```python
from build123d import *

# Parameters (mm, degrees)
F1_DEPTH = 76.708
F2_DEPTH = 77.47
F3_DEPTH = 38.1


with BuildPart() as f1:
    # F0 (on Top) → F1 (new body)
    with BuildSketch(Plane.XY):
        Polygon((135.3836357594, 21.8498203903), (-49.6764220297, -59.8627962172), (146.1022645235, -72.4891498685), align=None)
    extrude(amount=F1_DEPTH)

    # F2 (add): a face of the model
    f2_faces = [f1.faces().sort_by_distance(p)[0] for p in [
        (140.7429501414, -25.3196647391, 38.354),
    ]]
    extrude(f2_faces, amount=F2_DEPTH)

    # F3 (add): a face of the model
    f3_faces = [f1.faces().sort_by_distance(p)[0] for p in [
        (122.6602477732, -29.7614131006, 76.708),
    ]]
    extrude(f3_faces, amount=F3_DEPTH)


solid = f1.part
```
Source: CAD feature listing. Evaluate the final solid. Frame: model axes, mm. Round coordinates to 2 decimals unless told otherwise and drop trailing zeros. Order: outer loops, then holes, each group sorted by start corner. A loop starts at its lowest first (then second) coordinate and runs counter-clockwise, first axis right, second up. Notation, with made-up numbers: (15, 47) -> (27, 47) arc R25 cw to (27, 82) -> close; hole circle Ø2 at (21, 38). An arc over 180 degrees is marked (long way). One line per item, written item: value. Start each with the question number.
Q1. Section query C-C (x = 33.5). Return the cut outline in (y, z), plus the area to 3 significant figures.
Q2. Section query A-A (z = 83.5). Return the cut outline in (x, y).
Q3. Section query B-B (y = -20). Return the cut outline in (x, z).
Q4. Pin query (flat end, axial travel): pin 1 (6 mm diameter, centred on x = 112, z = 44.5, fed in from -Y); pin 2 (10 mm diameter, centred on x = 63.5, z = 38.5, fed in from -Y); pin 3 (2 mm diameter, centred on x = 97, z = 65, fed in from -Y). Return the tip coordinate at first contact, or that it passes through.
Q5. Material intervals for probe 1 along X at (y, z) = (-42, 95); probe 2 along X at (y, z) = (-35, 33.5); probe 3 along Y at (x, z) = (145, 13.5), sorted ascending.
Findings below:
1. outline: (-65.23, 0) -> (-23.14, 0) -> (-23.14, 114.81) -> (-65.23, 114.81) -> close
1. area: 4,830 mm²
2. outline: (-49.68, -59.86) -> (146.1, -72.49) -> (223.08, -63.74) -> (212.36, 30.6) -> (135.38, 21.85) -> close
3. outline: (40.6, 0) -> (218.11, 0) -> (218.11, 114.81) -> (40.6, 114.81) -> close
4. pin 1: y = -70.48
4. pin 2: y = -67.48
4. pin 3: y = -69.39
5. probe 1: -9.22 to 220.61
5. probe 2: 6.63 to 219.81
5. probe 3: -72.42 to 22.94
